Geometry: final body of the model. Coordinates: model frame, mm. A direction names the side the tool comes from. Round coordinates to 2 decimals unless told otherwise and drop trailing zeros. Write each loop counter-clockwise with the first axis right and the second up, starting at its lowest first coordinate (ties: lowest second). Pieces come first, ordered by that corner, then holes. Notation, with made-up numbers: M -29,-6.5 L 5,-6.5 A9 ccw 5,3.5 Z; hole C -39.5,14.5 d3. An arc over 180 degrees is marked long. Answer as CSV lines item,"result". Start each with the question number.
Q1. Section query A-A on z = 14.5. Output: boundary loops of the cut face in (x, y).
Q2. Reachability of faces 4 (the flat face through (-14.602, 5, 37)), 5 (the cylindrical face through (-14.076, 4.933, 29.041)), 6 (the flat face through (-68.15, 3, 36)), 7 (the flat face through (-80.213, 3, 10)) from +Z, -Z, +X, -X, +Y, -Y: full face, straight path, thin tool, end or side. Return the list, or none.
Q3. Section query B-B on y = 5. Output: boundary loops of the cut face in (x, z), and give its area (3 significant figures).
Q4. Mould query, pull axis X, two halves, no side actions, for faces 1 (the cylindrical face through (-79.935, 3.131, 20.918)), 2 (the cylindrical face through (-0.263, 3.131, 20.888)), 3 (the cylindrical face through (-7.87, 2.83, 23.35)). Classes: pulls with the +X half, pulls with the -X half, needs draft (parallel to the pull), parting line crosses it, or undercut.
Q5. First-contact query: pin 1 (2 mm diameter, centred on y = 3, z = 29.5, fed in from +X); pin 2 (1.3 mm diameter, centred on x = -22, z = 36, fed in from +Y); pin 3 (2 mm diameter, centred on y = 3.5, z = 35.5, fed in from +X); pin 4 (1 mm diameter, centred on x = -49, y = 5, fed in from +Z). Flat tips, straight axial feed; report the tip coordinate or a pass-through.
Q6. Ray query, probe 1 along X at (y, z) = (3.5, 4); probe 2 along X at (y, z) = (3.5, 32); probe 3 along X at (y, z) = (1.25, 33). Return the intervals inside material, ascending.
Q7. Section query D-D on z = 32.5. Output: boundary loops of the cut face in (x, y), and give its area (3 significant figures).
Q8. Section query C-C on x = -54.5. Output: boundary loops of the cut face in (y, z), and give its area (3 significant figures).
```python
from build123d import *

# Parameters (mm, degrees)
EXTRUDE1_DEPTH = 6.35
SHELL1_START   = 2.54
SHELL1_DEPTH   = 3.81
FILLET2_R      = 1.016
EXTRUDE2_DEPTH = 0.762
EXTRUDE2_TAPER = 25


# Read off the part's stored shape, not the designer's step: Shell1
with BuildPart() as part:
    # Sketch1 → Extrude1 (new body)
    with BuildSketch(Plane(origin=(0, 0, 0), x_dir=(1, 0, 0), z_dir=(0, 1, 0))):
        with BuildLine():
            Line((-14.602264877, -43.480257116), (-65.610482537, -43.480257116))
            ThreePointArc((-65.610482537, -43.480257116), (-67.406533761, -42.73630834), (-68.150482537, -40.940257116))
            Line((-68.150482537, -40.940257116), (-68.150482537, -31.291332317))
            ThreePointArc((-68.150482537, -31.291332317), (-68.420760673, -30.151173267), (-69.174075183, -29.253659935))
            Line((-69.174075183, -29.253659935), (-79.189154769, -21.800577453))
            ThreePointArc((-79.189154769, -21.800577453), (-79.942469279, -20.903064121), (-80.212747415, -19.762905071))
            Line((-80.212747415, -19.762905071), (-80.212747415, 0))
            Line((-80.212747415, 0), (0, 0))
            Line((0, 0), (0, -19.762905071))
            ThreePointArc((0, -19.762905071), (-0.270278136, -20.903064121), (-1.023592646, -21.800577453))
            Line((-1.023592646, -21.800577453), (-11.038672231, -29.253659935))
            ThreePointArc((-11.038672231, -29.253659935), (-11.791986741, -30.151173267), (-12.062264877, -31.291332317))
            Line((-12.062264877, -31.291332317), (-12.062264877, -40.940257116))
            ThreePointArc((-12.062264877, -40.940257116), (-12.806213653, -42.73630834), (-14.602264877, -43.480257116))
        make_face()
    extrude(amount=EXTRUDE1_DEPTH)

    # Shell1 outline → Shell1 (cut)
    with BuildSketch(Plane(origin=(0, 0, 0), x_dir=(1, 0, 0), z_dir=(0, 1, 0)).offset(SHELL1_START)):
        with BuildLine():
            Line((-14.602264877, -43.480257116), (-14.602264877, -31.291332317))
            ThreePointArc((-14.602264877, -31.291332317), (-14.061708605, -29.011014216), (-12.555079586, -27.215987553))
            Line((-12.555079586, -27.215987553), (-2.54, -19.762905071))
            Line((-2.54, -19.762905071), (-2.54, 0))
            Line((-2.54, 0), (-77.672747415, 0))
            Line((-77.672747415, 0), (-77.672747415, -19.762905071))
            Line((-77.672747415, -19.762905071), (-67.657667829, -27.215987553))
            ThreePointArc((-67.657667829, -27.215987553), (-66.151038809, -29.011014216), (-65.610482537, -31.291332317))
            Line((-65.610482537, -31.291332317), (-65.610482537, -43.480257116))
            Line((-65.610482537, -43.480257116), (-14.602264877, -43.480257116))
        make_face()
    extrude(amount=SHELL1_DEPTH, mode=Mode.SUBTRACT)

    # Fillet2
    fillet2_edges = [part.edges().sort_by_distance(p)[0] for p in [
        (-14.602264877, 2.54, 37.385794717),
        (-14.061708605, 2.54, 29.011014216),
        (-7.547539793, 2.54, 23.489446312),
        (-2.54, 2.54, 9.881452535),
        (-2.54, 4.445, 19.762905071),
        (-77.672747415, 2.54, 9.881452535),
        (-72.665207622, 2.54, 23.489446312),
        (-77.672747415, 4.445, 19.762905071),
        (-66.151038809, 2.54, 29.011014216),
        (-65.610482537, 2.54, 37.385794717),
    ]]
    fillet(fillet2_edges, radius=FILLET2_R)

    # Sketch3 → Extrude2 (add)
    with BuildSketch(Plane(origin=(0, 2.54, 0), x_dir=(-1, 0, 0), z_dir=(0, 1, 0))):
        Polygon((22.356461774, 33.449057502), (23.555013556, 36.122749938), (22.356461774, 38.796442374), (21.157909992, 36.122749938), align=None)
    extrude(amount=EXTRUDE2_DEPTH, taper=EXTRUDE2_TAPER)


solid = part.part
```
Entries:
1,outline,"M -80.21,0 L 0,0 L 0,6.35 L -2.54,6.35 L -2.54,3.56 A1.02 cw -3.56,2.54 L -76.66,2.54 A1.02 cw -77.67,3.56 L -77.67,6.35 L -80.21,6.35 Z"
2,face 4,"+Z, -Z, +Y"
2,face 5,"-Z, +Y"
2,face 6,"+Z, -X, +Y, -Y"
2,face 7,"+Z, -Z, -X, +Y, -Y"
3,outline,"M -80.21,0 L -77.67,0 L -77.67,19.25 A1.02 cw -77.26,20.07 L -67.66,27.22 A5.08 ccw -65.61,31.29 L -65.61,43.48 A2.54 ccw -68.15,40.94 L -68.15,31.29 A2.54 cw -69.17,29.25 L -79.19,21.8 A2.54 ccw -80.21,19.76 Z; M -14.6,31.29 A5.08 ccw -12.56,27.22 L -2.95,20.07 A1.02 cw -2.54,19.25 L -2.54,0 L 0,0 L 0,19.76 A2.54 ccw -1.02,21.8 L -11.04,29.25 A2.54 cw -12.06,31.29 L -12.06,40.94 A2.54 ccw -14.6,43.48 Z"
3,area,"247 mm^2"
4,face 1,"pulls with the -X half"
4,face 2,"pulls with the +X half"
4,face 3,"undercut"
5,pin 1,"stops at x = -10.03"
5,pin 2,"stops at y = 3.3"
5,pin 3,"stops at x = -12.06"
5,pin 4,"passes through"
6,probe 1,"x = -80.21 to -77.67, -2.54 to 0"
6,probe 2,"x = -68.15 to -65.61, -14.6 to -12.06"
6,probe 3,"x = -68.15 to -12.06"
7,outline,"M -68.15,0 L -12.06,0 L -12.06,6.35 L -14.6,6.35 L -14.6,3.56 A1.02 cw -15.62,2.54 L -64.59,2.54 A1.02 cw -65.61,3.56 L -65.61,6.35 L -68.15,6.35 Z"
7,area,"162 mm^2"
8,outline,"M 0,0 L 2.54,0 L 2.54,43.48 L 0,43.48 Z"
8,area,"110 mm^2"
